Autodesk Inventor part; units mm, degrees
ref_plane "YZ Plane" through (0, 0, 0) normal (1, 0, 0) x (0, 1, 0)
ref_plane "XZ Plane" through (0, 0, 0) normal (0, 1, 0) x (-1, 0, 0)
ref_plane "XY Plane" through (0, 0, 0) normal (0, 0, 1) x (1, 0, 0)
sketch "Skizze1" plane through (0, 0, 0) normal (0, 0, 1) x (1, 0, 0)
  line L0 (-2.5, 0) -> (5.5, 0)
  line L1 (9, 4.85) -> (9, 7.5)
  line L2 (9, 7.5) -> (2, 7.5)
  line L3 (-3, 4.85) -> (-3, 9)
  line L4 (-3, 9) -> (0, 9)
  line L5 (2, 7.5) -> (1.3299, 7.3204)
  line L6 (1.1746, 7.3) -> (0.5, 7.3)
  line L7 (-0.0869, 8.0247) -> (0, 8.4335)
  line L8 (0, 8.4335) -> (0, 9)
  arc A0 (-0.0869, 8.0247) -> (0.5, 7.3) centre (0.5, 7.9) ccw
  arc A1 (1.1746, 7.3) -> (1.3299, 7.3204) centre (1.1746, 7.9) ccw
  line L9 (-28.4, 0) -> (128.4, 0)
  line L10 (0, -12) -> (0, 72)
  line L11 (-3, 4.85) -> (9, 4.85)
  dimension "d0" = 18
  dimension "d1" = 15
  dimension "d2" = 12
  dimension "d3" = 12
  dimension "d4" = 0.6
  dimension "d5" = 0.1
  dimension "d6" = 2
  dimension "d7" = 15
  dimension "d8" = 0.2
  dimension "d9" = 0.6
  dimension "d10" = 3
  dimension "d11" = 9.7
revolve "Körper" add sketch "Skizze1" angle 360 about axis through (-2.5, 0, 0) along (1, 0, 0) contours L11 L10 A0 L6 A1 L5 L2 L1 | L11 L3 L4 L8 L7 A0 L10
chamfer "Fase1" distance 1.5 angle 15 1 edges at (9, -7.5, 0) measured on face at (6.6667, 7.4029, -1.2031)
fillet "Rundung1" radius 2 1 edges at (-3, -4.85, 0)
equation "\"d12\" = PHH"
equation "\"d13\" = ANG"
equation "\"d29\" = PHH"
equation "\"d14\" = RR"
equation "\"d0\" = KOD"
equation "\"d1\" = SD2"
equation "\"d2\" = NLG"
equation "\"d4\" = FSRR"
equation "\"d5\" = FST2"
equation "\"d6\" = FSB"
equation "\"d8\" = FST1"
equation "\"d9\" = FSRR"
equation "\"d10\" = KOH"
equation "\"d11\" = NND"
equation "\"NLG\" = 12"
equation "\"NND\" = 9.7"
equation "\"KOD\" = 18"
equation "\"KOH\" = 3"
equation "\"SD2\" = 15"
equation "\"FST1\" = 0.2"
equation "\"FST2\" = 0.1"
equation "\"FSB\" = 2"
equation "\"FSRR\" = 0.6"
equation "\"PHH\" = 1.5"
equation "\"ANG\" = 15deg"
equation "\"RR\" = 2"
equation "\"NNDMIN\" = 8.1"
equation "\"FSH\" = 1.4"
equation "\"SEWI\" = 30deg"
properties part number "DIN 172 - A 9,7 x 12" material "Stahl, weich"
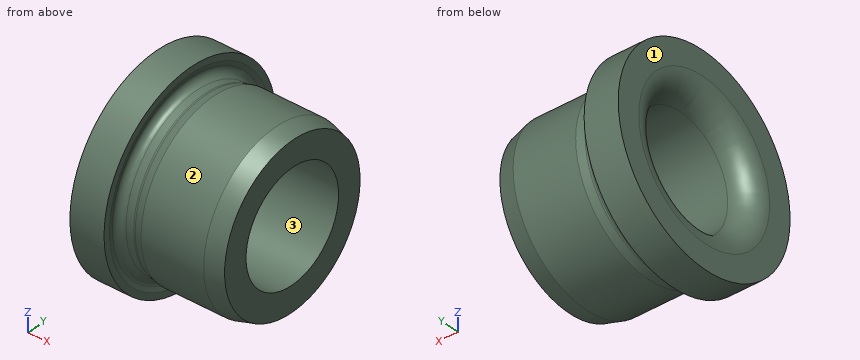
Input: part model. Units: mm. Frame: model coordinates. Face numbers are marked on the shaded views. Give positions to 0.01 mm unless a question says otherwise; leave off trailing zeros. Order: outer loops, then holes, each group sorted by start corner. A loop starts at its lowest first (then second) coordinate and runs counter-clockwise, first axis right, second up. Notation, with made-up numbers: M 59.5,59 L 69.5,59 A32 cw 69.5,91 Z; hole C 88.25,52 d3. An arc over 180 degrees is marked long. Return JSON: item names as keys, results as strings.
Item 1: Cut plane A-A (y = 0). Return loops of the section in (x, z), then the cut area to 3 significant figures.
Solutions:
{"outline": "M -3,-9 L 0,-9 L 0,-8.43 L -0.09,-8.02 A0.6 cw 0.5,-7.3 L 1.17,-7.3 A0.6 cw 1.33,-7.32 L 2,-7.5 L 7.5,-7.5 L 9,-7.1 L 9,-4.85 L -1,-4.85 A2 ccw -3,-6.85 Z; M -3,6.85 A2 ccw -1,4.85 L 9,4.85 L 9,7.1 L 7.5,7.5 L 2,7.5 L 1.33,7.32 A0.6 cw 1.17,7.3 L 0.5,7.3 A0.6 cw -0.09,8.02 L 0,8.43 L 0,9 L -3,9 Z", "area": "69.6 mm^2"}
Item 2: Cut plane C-C (x = -0.5). Return loops of the section in (y, z), then the cut area to 3 significant figures.
Solutions:
{"outline": "C 0,0 d18; hole C 0,0 d9.7", "area": "181 mm^2"}
Item 3: Ray query, probe 1 along Z at (x, y) = (3.5, 0); probe 2 along Y at (x, z) = (8.75, 3); probe 3 along Y at (x, z) = (-2, -4.5). Return the intervals inside material, ascending.
Solutions:
{"probe 1": "-7.5 to -4.85, 4.85 to 7.5", "probe 2": "-6.51 to -3.81, 3.81 to 6.51", "probe 3": "-7.79 to -2.44, 2.44 to 7.79"}
Item 4: First-contact query: P1, Ø3, axis at x = 5.5, y = -2.5, coming from the -Z side; P2, Ø3, axis at x = 2, z = 6, coming from the +Y side; P3, Ø4, axis at x = -1.5, y = 6, coming from the +Z side; P4, Ø8.5, axis at y = 0, z = 0, coming from the +X side. Flat tips, straight axial feed; report the tip coordinate or a pass-through.
Solutions:
{"P1": "z = -7.43", "P2": "y = 6", "P3": "z = 8.06", "P4": "through"}
Item 5: Pull-direction query (Y, two-part tool) for the marked faces 1, 2 and 3; classes: +Y half, -Y half, draft (parallel to the pull), parting line (faces both ways), or undercut.
Solutions:
{"face 1": "draft", "face 2": "parting line", "face 3": "undercut"}
Item 6: Cut plane D-D (x = 3). Return loops of the section in (y, z), then the cut area to 3 significant figures.
Solutions:
{"outline": "C 0,0 d15; hole C 0,0 d9.7", "area": "103 mm^2"}
